Autodesk Inventor part; units mm, degrees
ref_plane "YZ Plane" through (0, 0, 0) normal (1, 0, 0) x (0, 1, 0)
ref_plane "XZ Plane" through (0, 0, 0) normal (0, 1, 0) x (-1, 0, 0)
ref_plane "XY Plane" through (0, 0, 0) normal (0, 0, 1) x (1, 0, 0)
sketch "Skizze1" plane through (0, 0, 0) normal (0, 0, 1) x (1, 0, 0)
  line L0 (-175, 0) -> (175, 0) construction
  line L1 (0, 21) -> (0, -21) construction
  line L2 (-125, -15) -> (125, -15)
  line L3 (125, -15) -> (125, 15)
  line L4 (125, 15) -> (-125, 15)
  line L5 (-125, 15) -> (-125, -15)
  line L6 (-125, -15) -> (125, 15) construction
  line L7 (125, -15) -> (-125, 15) construction
  point P0 (0, 0)
  dimension "d0" = 250
  dimension "d1" = 30
extrude "Grundkörper" add sketch "Skizze1" along normal mid plane 15
sketch "Skizze2" plane through (0, 0, 7.5) normal (0, 0, 1) x (1, 0, 0)
  line L0 (0, 21) -> (0, -21) construction
  point P0 (0, 0)
  point P1 (-115.6, 0)
  point P2 (115.6, 0)
  dimension "d4" = 231.2
hole "M6" at (-115.6, 0, 7.5) at (115.6, 0, 7.5) direction (0, 0, -1) diameter 4.917 end through all
sketch "Skizze3" plane through (0, 0, 7.5) normal (0, 0, 1) x (1, 0, 0)
  line L0 (0, 21) -> (0, -21) construction
  line L1 (-97.5, 7.5) -> (-27.5, 7.5)
  line L2 (-22.5, 2.5) -> (-22.5, -2.5)
  line L3 (-27.5, -7.5) -> (-97.5, -7.5)
  line L4 (-102.5, -2.5) -> (-102.5, 2.5)
  line L5 (-175, 0) -> (175, 0) construction
  line L6 (125, 15) -> (-125, 15)
  line L7 (0, 15) -> (-125, 15)
  line L8 (-62.5, 15) -> (-62.5, -15) construction
  line L9 (-125, -15) -> (125, -15) construction
  arc A0 (-102.5, -2.5) -> (-97.5, -7.5) centre (-97.5, -2.5) ccw
  arc A1 (-97.5, 7.5) -> (-102.5, 2.5) centre (-97.5, 2.5) ccw
  arc A2 (-22.5, 2.5) -> (-27.5, 7.5) centre (-27.5, 2.5) ccw
  arc A3 (-27.5, -7.5) -> (-22.5, -2.5) centre (-27.5, -2.5) ccw
  point P0 (0, 0)
  point P1 (-102.5, 7.5)
  point P2 (-22.5, 7.5)
  dimension "d16" = 15
  dimension "d17" = 80
  dimension "d18" = 5
extrude "Ausschnitt_Gewichtsreduktion" cut sketch "Skizze3" against normal through all
mirror "Spiegeln_Ausschnitt_Gewichtsreduktion" about plane through (0, 0, 0) normal (1, 0, 0) of "Ausschnitt_Gewichtsreduktion"
chamfer "Fase_M6_Gewinde" distance 0.5 angle 45 4 edges at (-115.6, 2.4585, -7.5) (115.6, 2.4585, -7.5) (-115.6, 2.4585, 7.5) (115.6, 2.4585, 7.5)
sketch "Skizze4" plane through (0, 0, 7.5) normal (0, 0, 1) x (1, 0, 0)
  line L0 (0, 21) -> (0, -21) construction
  line L1 (-175, 0) -> (175, 0) construction
  point P0 (0, 0)
  point P1 (0, 0)
hole "12H7_Bohrung" at (0, 0, 7.5) direction (0, 0, -1) diameter 12 end through all
fillet "Abrundung" radius 10 4 edges at (-125, 15, 0) (-125, -15, 0) (125, -15, 0) (125, 15, 0)
chamfer "Fase_Allgemein" distance 2 angle 45 8 edges at (0, -15, 7.5) (122.0711, -12.0711, 7.5) (0, 15, 7.5) (-122.0711, 12.0711, 7.5) (0, -15, -7.5) (-122.0711, 12.0711, -7.5) (0, 15, -7.5) (122.0711, -12.0711, -7.5)
chamfer "Fase_Bohrung" distance 1 angle 45 2 edges at (0, 6, 7.5) (0, 6, -7.5)
properties part number "200-60-DIFFERENTIAL-CONNECTOR-01" material "Edelstahl"
Work out the finished part from the listing and answer in its coordinate system (mm). A direction names the side the tool comes from. Round coordinates to 2 decimals unless told otherwise and drop trailing zeros. Write each loop counter-clockwise with the first axis right and the second up, starting at its lowest first coordinate (ties: lowest second). Pieces come first, ordered by that corner, then holes. Notation, with made-up numbers: (8, 72) -> (54, 72) arc R17 cw to (54, 81) -> close; hole circle Ø9 at (57.5, 85). An arc over 180 degrees is marked (long way). Write each question's results on one line, items separated by ' | '.
Item 1: A cutting plane is placed at C-C, the plane x = 72.5. Determine the outline of the cut face in (y, z).
Result set:
outline: (-15, -5.5) -> (-13, -7.5) -> (-7.5, -7.5) -> (-7.5, 7.5) -> (-13, 7.5) -> (-15, 5.5) -> close; (7.5, -7.5) -> (13, -7.5) -> (15, -5.5) -> (15, 5.5) -> (13, 7.5) -> (7.5, 7.5) -> close
Item 2: Find the intervals of material crossed by line 1 along X through (y, z) = (0, -0.25); line 2 along Y through (x, z) = (78.5, 2.5); line 3 along Y through (x, z) = (115.6, 0.75), in increasing order. Write a range as [from, to].
Result set:
line 1: [-125, -118.06], [-113.14, -102.5], [-22.5, -6], [6, 22.5], [102.5, 113.14], [118.06, 125] | line 2: [-15, -7.5], [7.5, 15] | line 3: [-14.98, -2.46], [2.46, 14.98]
Item 3: A cutting plane is placed at D-D, the plane y = 0. Count the separate pieces of the cut face and the enclosed holes in it, plus the area to 3 significant figures.
Result set:
separate pieces: 6 | enclosed holes: 0 | area: 1,010 mm^2
Item 4: The mould has two halves that part along Y. Classify faces 1 (the face through (-102.5, 0, 0)), 2 (the face through (-2, -15, 0)), 3 (the face through (121.13, 10.99, -6.93)): +Y half, -Y half, draft (parallel to the pull), parting line (faces both ways), or undercut.
Result set:
face 1: undercut | face 2: -Y half | face 3: +Y half
Item 5: Which of the six approach directions +Z, -Z, +X, -X, +Y, -Y give full straight-line access (tool end or side, diameter ignored) to faces 4 (the face through (101.07, 6, 0.11)), 5 (the face through (120.99, 11.13, 6.93))?
Result set:
face 4: +Z, -Z | face 5: +Z, +X, +Y
Item 6: A cutting plane is placed at A-A, the plane x = 0. Determine the outline of the cut face in (y, z), plus the area to 3 significant figures.
Result set:
outline: (-15, -5.5) -> (-13, -7.5) -> (-7, -7.5) -> (-6, -6.5) -> (-6, 6.5) -> (-7, 7.5) -> (-13, 7.5) -> (-15, 5.5) -> close; (6, -6.5) -> (7, -7.5) -> (13, -7.5) -> (15, -5.5) -> (15, 5.5) -> (13, 7.5) -> (7, 7.5) -> (6, 6.5) -> close | area: 260 mm^2
Item 7: Flat-ended cylindrical pins translate along their axes: P1, Ø2, axis at y = 8.5, z = -3.5, coming from the -X side; P2, Ø6, axis at y = 10, z = 3.5, coming from the +X side; P3, Ø6, axis at y = -11, z = -2.5, coming from the -X side. Find the tip coordinate at first contact, or state that the pin passes through.
Result set:
P1: x = -124.68 | P2: x = 124.8 | P3: x = -124.54
Item 8: A cutting plane is placed at B-B, the plane z = 1. Determine the outline of the cut face in (x, y), plus the area to 3 significant figures.
Result set:
outline: (-125, -5) arc R10 ccw to (-115, -15) -> (115, -15) arc R10 ccw to (125, -5) -> (125, 5) arc R10 ccw to (115, 15) -> (-115, 15) arc R10 ccw to (-125, 5) -> close; hole circle Ø4.92 at (-115.6, 0); hole (-102.5, -2.5) arc R5 ccw to (-97.5, -7.5) -> (-27.5, -7.5) arc R5 ccw to (-22.5, -2.5) -> (-22.5, 2.5) arc R5 ccw to (-27.5, 7.5) -> (-97.5, 7.5) arc R5 ccw to (-102.5, 2.5) -> close; hole circle Ø12 at (0, 0); hole (22.5, -2.5) arc R5 ccw to (27.5, -7.5) -> (97.5, -7.5) arc R5 ccw to (102.5, -2.5) -> (102.5, 2.5) arc R5 ccw to (97.5, 7.5) -> (27.5, 7.5) arc R5 ccw to (22.5, 2.5) -> close; hole circle Ø4.92 at (115.6, 0) | area: 4,910 mm^2
